Could you check a few things on this model? Use its own coordinates, in mm. A direction names the side the tool comes from. Round coordinates to 2 decimals unless told otherwise and drop trailing zeros. Loops run counter-clockwise (first coordinate to the right, second up) from the corner with the lowest first, then second, coordinate; pieces in that order, holes last. Notation, with made-up numbers: (39, 23.5) -> (80, 23.5) arc R29 ccw to (80, 59.5) -> close; hole circle Ø8 at (39.25, 50). An arc over 180 degrees is marked (long way). One line per item, written item: value.
```python
from build123d import *

# Parameters (mm, degrees)
SKETCH2_R           = 11
SKETCH2_R_2         = 2
SKETCH2_R_3         = 1.244152151
BOSS_EXTRUDE1_DEPTH = 3
SKETCH3_R           = 5
SKETCH3_R_2         = 2
BOSS_EXTRUDE3_DEPTH = 10
CUT_EXTRUDE2_START  = 5
SKETCH6_R           = 1.875
CUT_EXTRUDE2_DEPTH  = 3.2
SKETCH10_R          = 1.5
CUT_EXTRUDE3_DEPTH  = 3


with BuildPart() as part:
    # Sketch2 → Boss-Extrude1 (new body)
    with BuildSketch(Plane.XY):
        Circle(SKETCH2_R)
        Circle(SKETCH2_R_2, mode=Mode.SUBTRACT)
        with Locations((-5.656854249, 5.656854249)):
            Circle(SKETCH2_R_3, mode=Mode.SUBTRACT)
        with Locations((5.656854249, 5.656854249)):
            Circle(SKETCH2_R_3, mode=Mode.SUBTRACT)
        with Locations((5.656854249, -5.656854249)):
            Circle(SKETCH2_R_3, mode=Mode.SUBTRACT)
        with Locations((-5.656854249, -5.656854249)):
            Circle(SKETCH2_R_3, mode=Mode.SUBTRACT)
    extrude(amount=BOSS_EXTRUDE1_DEPTH)

    # Sketch3 → Boss-Extrude3 (add)
    with BuildSketch(Plane.XY.offset(3)):
        Circle(SKETCH3_R)
        Circle(SKETCH3_R_2, mode=Mode.SUBTRACT)
    extrude(amount=BOSS_EXTRUDE3_DEPTH)

    # Sketch6 → Cut-Extrude2 (cut)
    with BuildSketch(Plane(origin=(0, 0, 0), x_dir=(1, 0, 0), z_dir=(0, 1, 0)).offset(CUT_EXTRUDE2_START)):
        with Locations(Location((0, -7.5, 0), (0, 0, 270))):
            Circle(SKETCH6_R)
    extrude(amount=-CUT_EXTRUDE2_DEPTH, mode=Mode.SUBTRACT)

    # Sketch10 → Cut-Extrude3 (cut)
    with BuildSketch(Plane(origin=(0, 0, 0), x_dir=(1, 0, 0), z_dir=(0, 1, 0))):
        with Locations((0, -7.5)):
            Circle(SKETCH10_R)
    extrude(amount=CUT_EXTRUDE3_DEPTH, mode=Mode.SUBTRACT)


solid = part.part
```
(1) Please list where these lines run through material, in increasing order: L1, parallel to Z at x = 0, y = 3.8 (3 decimals); L2, parallel to Y at x = 0, z = 10.75; L3, parallel to Z at x = 6.75, y = 0.5.
Results below:
L1: z = 0 to 5.625, 9.375 to 13
L2: y = -5 to -2, 2 to 5
L3: z = 0 to 3
(2) Imagine slicing it at D-D on x = 3.5. Write out the boundary of the cut face in (y, z).
Results below:
outline: (-10.43, 0) -> (10.43, 0) -> (10.43, 3) -> (3.57, 3) -> (3.57, 13) -> (-3.57, 13) -> (-3.57, 3) -> (-10.43, 3) -> close
(3) Imagine slicing it at A-A on y = 0. Write out the boundary of the cut face in (x, z).
Results below:
outline: (-11, 0) -> (-2, 0) -> (-2, 13) -> (-5, 13) -> (-5, 3) -> (-11, 3) -> close; (2, 0) -> (11, 0) -> (11, 3) -> (5, 3) -> (5, 13) -> (2, 13) -> close
(4) For pin 1 Ø2 at (x, z) = (-1.5, 9.5) entering from +Y; pin 2 Ø4 at (x, z) = (-2.5, 11) entering from -Y; pin 3 Ø2 at (x, y) = (-5.66, -5.66) entering from +Z; pin 4 Ø0.5 at (x, z) = (-1, 8) entering from +Y, each with a flat end and sliding along its axis, tell me the tip position at first contact or that it passes through.
Results below:
pin 1: stops at y = 4.97
pin 2: stops at y = -4.97
pin 3: passes through
pin 4: stops at y = -1.56
(5) We'd pull the mould along Z, two halves only. Please class faces 1 (the face through (6.844, 6.031, 1.479)), 2 (the face through (-1.7, 1.8, 7.5)), 3 (the face through (-0.2, -2.3, 0)): +Z half, -Z half, draft (parallel to the pull), parting line (faces both ways), or undercut.
Results below:
face 1: draft
face 2: undercut
face 3: -Z half
(6) Imagine slicing it at C-C on z = 7.25. Write out the boundary of the cut face in (x, y), then the cut area to 3 significant figures.
Results below:
outline: (-1.86, 1.8) -> (-1.86, 4.64) arc R5 ccw (long way) to (1.86, 4.64) -> (1.86, 1.8) -> (1.48, 1.8) -> (1.48, 1.35) arc R2 cw (long way) to (-1.48, 1.35) -> (-1.48, 1.8) -> close
area: 54.5 mm²
(7) On a 3-axis mill with a long thin cutter (end or side, diameter ignored), from which of +Z, -Z, +X, -X, +Y, -Y can I reach the whole of each face in a straight line? I mean faces 4 (the face through (-6.574, -4.816, 1.479)), 5 (the face through (5, -2, 3)), 6 (the face through (-1.83, 3.42, 7.09)). Say none if no direction works.
Results below:
face 4: +Z, -Z
face 5: +Z
face 6: +Y
(8) Imagine slicing it at B-B on x = 0. Write out the boundary of the cut face in (y, z) (3 decimals), then the cut area to 3 significant figures.
Results below:
outline: (-11, 0) -> (-2, 0) -> (-2, 13) -> (-5, 13) -> (-5, 3) -> (-11, 3) -> close; (2, 0) -> (11, 0) -> (11, 3) -> (5, 3) -> (5, 5.625) -> (2, 5.625) -> close; (2, 9.375) -> (5, 9.375) -> (5, 13) -> (2, 13) -> close
area: 103 mm²
